from build123d import *

# Parameters (mm, degrees)
SKETCH1_W        = 101.6
SKETCH1_H        = 76.2
BODY_DEPTH       = 38.1
CORNER_FILLETS_R = 6.35
SHELL_T          = -2.54
CABLE_HOLE_REACH = 117.003
SKETCH2_R        = 6.307285196


with BuildPart() as part:
    # Sketch1 → Body (new body)
    with BuildSketch(Plane(origin=(0, 0, 0), x_dir=(1, 0, 0), z_dir=(0, 1, 0))):
        Rectangle(SKETCH1_W, SKETCH1_H)
    extrude(amount=BODY_DEPTH)

    # Corner Fillets
    corner_fillets_edges = [part.edges().sort_by_distance(p)[0] for p in [
        (50.8, 19.05, 38.1),
        (-50.8, 19.05, 38.1),
        (-50.8, 19.05, -38.1),
        (50.8, 19.05, -38.1),
    ]]
    fillet(corner_fillets_edges, radius=CORNER_FILLETS_R)

    # Shell
    shell_openings = [part.faces().sort_by_distance(p)[0] for p in [
        (0, 38.1, 0),
    ]]
    offset(amount=SHELL_T, openings=shell_openings, kind=Kind.INTERSECTION)

    # Sketch2 → Cable Hole (cut, up to next)
    with BuildSketch(Plane.ZY.offset(50.8), mode=Mode.PRIVATE) as cable_hole_sk1:
        with Locations((0, 19.085434186)):
            Circle(SKETCH2_R)
    cable_hole_tool1 = extrude(cable_hole_sk1.sketch, amount=-CABLE_HOLE_REACH, mode=Mode.PRIVATE) & part.part
    add(cable_hole_tool1.solids().sort_by_distance((-50.8, 19.085434, 0))[0], mode=Mode.SUBTRACT)


solid = part.part
Geometry check sheet. Reference: the model listing, model coordinates, mm. A direction names the side the tool comes from. Give positions to 0.01 mm unless a question says otherwise; leave off trailing zeros. Order: outer loops, then holes, each group sorted by start corner. A loop starts at its lowest first (then second) coordinate and runs counter-clockwise, first axis right, second up.
1. Sectioned sample at C-C (x = 40.5). Record the boundary of the cut face in (y, z), then the cut area to 3 significant figures.
Completed:
outline: (0, -38.1) - (38.1, -38.1) - (38.1, -35.56) - (2.54, -35.56) - (2.54, 35.56) - (38.1, 35.56) - (38.1, 38.1) - (0, 38.1) - close
area: 374 mm2
2. Sectioned sample at A-A (z = 0). Record the boundary of the cut face in (x, y).
Completed:
outline: (-50.8, 0) - (50.8, 0) - (50.8, 38.1) - (48.26, 38.1) - (48.26, 2.54) - (-48.26, 2.54) - (-48.26, 12.78) - (-50.8, 12.78) - close; (-50.8, 25.39) - (-48.26, 25.39) - (-48.26, 38.1) - (-50.8, 38.1) - close
3. Sectioned sample at B-B (y = 31). Record the boundary of the cut face in (x, z), then the cut area to 3 significant figures.
Completed:
outline: (-50.8, -31.75) arc R6.35 ccw to (-44.45, -38.1) - (44.45, -38.1) arc R6.35 ccw to (50.8, -31.75) - (50.8, 31.75) arc R6.35 ccw to (44.45, 38.1) - (-44.45, 38.1) arc R6.35 ccw to (-50.8, 31.75) - close; hole (-48.26, -31.75) arc R3.81 ccw to (-44.45, -35.56) - (44.45, -35.56) arc R3.81 ccw to (48.26, -31.75) - (48.26, 31.75) arc R3.81 ccw to (44.45, 35.56) - (-44.45, 35.56) arc R3.81 ccw to (-48.26, 31.75) - close
area: 855 mm2
4. Depth check by flat-ended pin: pin 1 (5 mm diameter, centred on x = -0.5, z = 27.5, fed in from +Y). Enter the tip coordinate at first touch or a pass-through.
Completed:
pin 1: stops at y = 2.54
5. Scan lines: line 1 (Z direction, x = 3, y = 26.5); line 2 (Y direction, x = -49.3, z = 0); line 3 (X direction, y = 24, z = 10.5). Record each from-to range of solid material in increasing order.
Completed:
line 1: z = -38.1 to -35.56, 35.56 to 38.1
line 2: y = 0 to 12.78, 25.39 to 38.1
line 3: x = -50.8 to -48.26, 48.26 to 50.8
6. Access from +Z, -Z, +X, -X, +Y, -Y to the whole of each face (thin tool, end or side, straight path). Record for faces 5 (the face through (-49.548, 15.248, -5.005)), 6 (the face through (0, 38.1, -37)), 7 (the face through (-1, 20, 35.56)).
Completed:
face 5: -X
face 6: +Z, -Z, +X, -X, +Y
face 7: +Y
7. Draft check along Z on faces 1 (the face through (-48.99, 19.32, -36.19)), 2 (the face through (-1, 2.54, 0)), 3 (the face through (-47.174, 20.569, -34.414)), 4 (the face through (-50.8, 19, -7)). Enter one of: pulls with the +Z half, pulls with the -Z half, needs draft (parallel to the pull), parting line crosses it, or undercut.
Completed:
face 1: pulls with the -Z half
face 2: undercut
face 3: undercut
face 4: needs draft
